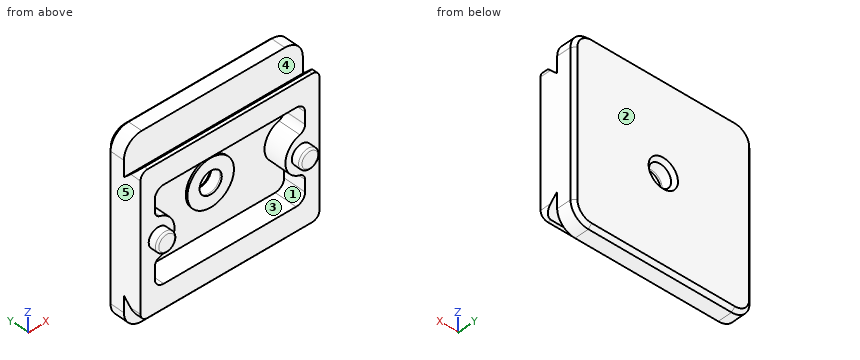
from build123d import *

# Parameters (mm, degrees)
SKETCH1_W           = 50
SKETCH1_H           = 50
BOSS_EXTRUDE1_DEPTH = 10
CUT_EXTRUDE3_DEPTH  = 6.3
SKETCH5_R           = 6.5
SKETCH5_R_2         = 3.1
BOSS_EXTRUDE2_DEPTH = 0.5
SKETCH6_R           = 2.7
BOSS_EXTRUDE3_DEPTH = 2.5
FILLET1_R           = 0.5
CUT_EXTRUDE4_DEPTH  = 57.789083458
FILLET2_R           = 5
CHAMFER1_SIZE       = 1
CHAMFER2_SIZE       = 1
CHAMFER2_SIZE2      = 1.414213562
FILLET3_R           = 2
SKETCH9_R           = 3.1
CUT_EXTRUDE5_DEPTH  = 37.434050008
CHAMFER3_SIZE       = 1


with BuildPart() as part:
    # Sketch1 → Boss-Extrude1 (new body)
    with BuildSketch(Plane(origin=(0, 0, 0), x_dir=(1, 0, 0), z_dir=(0, 1, 0))):
        Rectangle(SKETCH1_W, SKETCH1_H)
    extrude(amount=BOSS_EXTRUDE1_DEPTH)

    # Sketch4 → Cut-Extrude3 (cut)
    with BuildSketch(Plane(origin=(0, 0, 0), x_dir=(-1, 0, 0), z_dir=(0, -1, 0))):
        with BuildLine():
            Line((21, -7.228416147), (21, -10.5))
            ThreePointArc((21, -10.5), (20.267766953, -12.267766953), (18.5, -13))
            Line((18.5, -13), (-18.5, -13))
            ThreePointArc((-18.5, -13), (-20.267766953, -12.267766953), (-21, -10.5))
            Line((-21, -10.5), (-21, -7.228416147))
            ThreePointArc((-21, -7.228416147), (-20.591644852, -6.017356006), (-19.533333333, -5.300838508))
            ThreePointArc((-19.533333333, -5.300838508), (-15.5, 0), (-19.533333333, 5.300838508))
            ThreePointArc((-19.533333333, 5.300838508), (-20.591644852, 6.017356006), (-21, 7.228416147))
            Line((-21, 7.228416147), (-21, 10.5))
            ThreePointArc((-21, 10.5), (-20.267766953, 12.267766953), (-18.5, 13))
            Line((-18.5, 13), (18.5, 13))
            ThreePointArc((18.5, 13), (20.267766953, 12.267766953), (21, 10.5))
            Line((21, 10.5), (21, 7.228416147))
            ThreePointArc((21, 7.228416147), (20.591644852, 6.017356006), (19.533333333, 5.300838508))
            ThreePointArc((19.533333333, 5.300838508), (15.5, 0), (19.533333333, -5.300838508))
            ThreePointArc((19.533333333, -5.300838508), (20.591644852, -6.017356006), (21, -7.228416147))
        make_face()
    extrude(amount=-CUT_EXTRUDE3_DEPTH, mode=Mode.SUBTRACT)

    # Sketch5 → Boss-Extrude2 (add)
    with BuildSketch(Plane(origin=(0, 6.3, 0), x_dir=(-1, 0, 0), z_dir=(0, -1, 0))):
        with Locations(Location((0, 0, 0), (0, 0, 90))):
            Circle(SKETCH5_R)
        with Locations(Location((0, 0, 0), (0, 0, 90))):
            Circle(SKETCH5_R_2, mode=Mode.SUBTRACT)
    extrude(amount=BOSS_EXTRUDE2_DEPTH)

    # Sketch6 → Boss-Extrude3 (add)
    with BuildSketch(Plane.XZ):
        with Locations(Location((-20, 0, 0), (0, 0, 90))):
            Circle(SKETCH6_R)
        with Locations(Location((20, 0, 0), (0, 0, 90))):
            Circle(SKETCH6_R)
    extrude(amount=BOSS_EXTRUDE3_DEPTH)

    # Fillet1
    fillet1_edges = [part.edges().sort_by_distance(p)[0] for p in [
        (-20, -2.5, -2.7),
        (20, -2.5, -2.7),
    ]]
    fillet(fillet1_edges, radius=FILLET1_R)

    # Sketch8 → Cut-Extrude4 (cut, through all)
    with BuildSketch(Plane(origin=(25, 0, 0), x_dir=(0, 0, -1), z_dir=(1, 0, 0))):
        Polygon((-25, 0), (-25, 5), (-15.5, 5), (-20.5, 0), align=None)
        Polygon((25, 0), (25, 5), (15.5, 5), (20.5, 0), align=None)
    extrude(amount=-CUT_EXTRUDE4_DEPTH, mode=Mode.SUBTRACT)

    # Fillet2
    fillet2_edges = [part.edges().sort_by_distance(p)[0] for p in [
        (-25, 7.5, -25),
        (25, 7.5, -25),
        (25, 7.5, 25),
        (-25, 7.5, 25),
    ]]
    fillet(fillet2_edges, radius=FILLET2_R)

    # Chamfer1
    chamfer1_edges = [part.edges().sort_by_distance(p)[0] for p in [
        (0, 10, -25),
        (25, 10, 0),
        (-25, 10, 0),
        (0, 10, 25),
        (23.535533906, 10, 23.535533906),
        (-23.535533906, 10, 23.535533906),
        (-23.535533906, 10, -23.535533906),
        (23.535533906, 10, -23.535533906),
    ]]
    chamfer(chamfer1_edges, length=CHAMFER1_SIZE)

    # Chamfer2
    chamfer2_edges = [part.edges().sort_by_distance(p)[0] for p in [
        (0, 0, 20.5),
        (0, 0, -20.5),
    ]]
    chamfer2_side = [part.faces().sort_by_distance(p)[0] for p in [
        (24.353393474, 0, 0),
    ]]
    chamfer(chamfer2_edges, length=CHAMFER2_SIZE, length2=CHAMFER2_SIZE2, reference=chamfer2_side[0])

    # Fillet3
    fillet3_edges = [part.edges().sort_by_distance(p)[0] for p in [
        (25, 0.5, -19.5),
        (25, 0.5, 19.5),
        (-25, 0.5, -19.5),
        (-25, 0.5, 19.5),
    ]]
    fillet(fillet3_edges, radius=FILLET3_R)

    # Sketch9 → Cut-Extrude5 (cut, through all)
    with BuildSketch(Plane(origin=(0, 6.3, 0), x_dir=(-1, 0, 0), z_dir=(0, -1, 0))):
        with Locations(Location((0, 0, 0), (0, 0, 90))):
            Circle(SKETCH9_R)
    extrude(amount=-CUT_EXTRUDE5_DEPTH, mode=Mode.SUBTRACT)

    # Chamfer3
    chamfer3_edges = [part.edges().sort_by_distance(p)[0] for p in [
        (0, 10, 3.1),
    ]]
    chamfer(chamfer3_edges, length=CHAMFER3_SIZE)


solid = part.part
Build history of the part. All positions in model axes, mm. Face numbers are marked on the shaded views. A direction names the side the tool comes from. Coordinates: 2 decimals unless noted, no trailing zeros. Order: outer loops, then holes, each group sorted by start corner. A loop starts at its lowest first (then second) coordinate and runs counter-clockwise, first axis right, second up. Notation, with made-up numbers: M 18.5,-15 L 76.5,-15 A10 cw 76.5,-3 Z; hole C 60.5,-4 d4. An arc over 180 degrees is marked long. One line per question, with ' | ' between items. Start each with the question number.
Q1. Saw through at C-C (x = 0). List the corners of the cut face in (y, z).
Q2. Two-plate mould, pull along X, no slides. Class the marked faces 3, 4 and 5: +X half, -X half, draft (parallel to the pull), parting line (faces both ways), or undercut.
Q3. Saw through at D-D (x = 11). List the corners of the cut face in (y, z).
Q4. Probe L1, parallel to X at y = 6.15, z = 0; L2, parallel to X at y = 4.5, z = 9; L3, parallel to X at y = 8.3, z = 0. List the from-to ranges inside material, lowest first. Write a range as from..to.
Q5. 3-axis set-ups, long thin cutter, end or side, ignore diameter. For the marked faces 1 and 2: which of +Z, -Z, +X, -X, +Y, -Y reach the whole face in a straight line?
Q6. Saw through at B-B (y = 8.25). List the corners of the cut face in (x, z), then the cut area to 3 significant figures.
Q7. Flat gauge pins, fed straight in: pin 1 Ø4 at (x, z) = (0, -2) entering from -Y; pin 2 Ø19.5 at (x, z) = (3.5, 9.5) entering from -Y; pin 3 Ø3 at (x, z) = (-3.5, 8.5) entering from -Y; pin 4 Ø3.5 at (x, z) = (0, 0) entering from -Y. Where does each tip first touch, or does it go through?
Check values:
1) outline: M 0,-19.5 L 1,-19.5 L 5,-15.5 L 5,-25 L 9,-25 L 10,-24 L 10,-4.1 L 9,-3.1 L 5.8,-3.1 L 5.8,-6.5 L 6.3,-6.5 L 6.3,-13 L 0,-13 Z; M 0,13 L 6.3,13 L 6.3,6.5 L 5.8,6.5 L 5.8,3.1 L 9,3.1 L 10,4.1 L 10,24 L 9,25 L 5,25 L 5,15.5 L 1,19.5 L 0,19.5 Z
2) face 3: undercut | face 4: draft | face 5: -X half
3) outline: M 0,-19.5 L 1,-19.5 L 5,-15.5 L 5,-25 L 9,-25 L 10,-24 L 10,24 L 9,25 L 5,25 L 5,15.5 L 1,19.5 L 0,19.5 L 0,13 L 6.3,13 L 6.3,-13 L 0,-13 Z
4) L1: x = -25..-15.5, -6.5..-3.1, 3.1..6.5, 15.5..25 | L2: x = -25..-21, 21..25 | L3: x = -25..-3.1, 3.1..25
5) face 1: -Y | face 2: +Z, -Z, +X, -X, +Y
6) outline: M -25,-20 A5 ccw -20,-25 L 20,-25 A5 ccw 25,-20 L 25,20 A5 ccw 20,25 L -20,25 A5 ccw -25,20 Z; hole C 0,0 d6.2 | area: 2,450 mm2
7) pin 1: stops at y = 5.8 | pin 2: stops at y = 0 | pin 3: stops at y = 6.3 | pin 4: passes through
